The listing builds one solid part. Answer for the finished solid, in the listing's coordinates (mm). Face numbers are marked on the shaded views. A direction names the side the tool comes from. Round coordinates to 2 decimals unless told otherwise and drop trailing zeros. Order: outer loops, then holes, each group sorted by start corner. A loop starts at its lowest first (then second) coordinate and runs counter-clockwise, first axis right, second up. Notation, with made-up numbers: (74.5, 19.25) - (114.5, 19.25) arc R18 ccw to (114.5, 36.25) - close; hole circle Ø6 at (-32, 61.5). An arc over 180 degrees is marked (long way). Use CSV: the item, a comma, the result in double quotes. Start each with the question number.
Item 1: Find section C-C, the plane y = 29.5. Give the vertices of the cut face in (x, z), plus the area to 3 significant figures.
Item 2: Straight lines are drawn through the part: line 1 along X through (y, z) = (40, 0); line 2 along X through (y, z) = (2, -12.5); line 3 along X through (y, z) = (38.5, 6.5). For each, find the intervals that lie inside material, in ascending order. Write a range as [from, to].
Item 3: Flat-ended cylindrical pins translate along their axes: P1, Ø8, axis at x = -57, y = 34.5, coming from the -Z side; P2, Ø1.5, axis at x = -64.5, y = 41, coming from the +Z side; P3, Ø12, axis at y = 21, z = -34, coming from the +X side; P4, Ø9, axis at x = -61.25, z = 0, coming from the +Y side. Find the tip coordinate at first contact, or state that the pin passes through.
Item 4: Find section A-A, the plane x = 61.25. Give the vertices of the cut face in (y, z).
Item 5: Find section D-D, the plane y = 8. Give the vertices of the cut face in (x, z).
Item 6: For the marked faces 1, 2, 3, 4 and 5, determine the directions among +Z, -Z, +X, -X, +Y, -Y from which every point of the face is accessible in a straight line to the end or side of a thin tool.
Item 7: Find section B-B, the plane z = 0. Give the vertices of the cut face in (x, y).
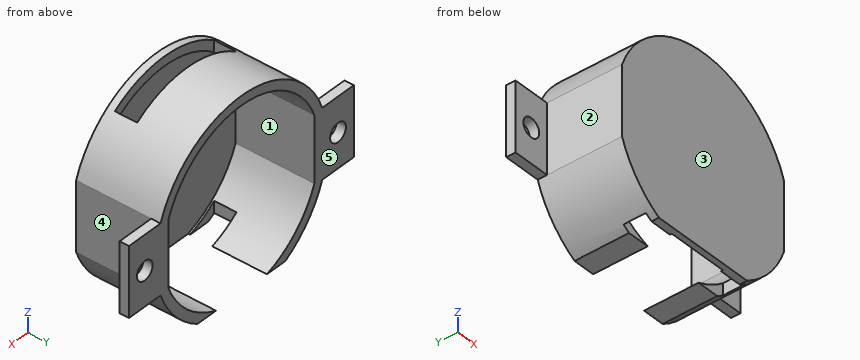
```python
from build123d import *

# Parameters (mm, degrees)
EXTRUDE_1_DEPTH          = 42.3
EXTRUDE_START            = 3
EXTRUDE_2_DEPTH          = 3
SKETCH_3_W               = 37.077621282
SKETCH_3_H               = 5
EXTRUDE_4_DEPTH          = 20
SKETCH_5_W               = 37.077621282
SKETCH_5_H               = 5
EXTRUDE_5_DEPTH          = 20
CUT_EXTRUDE_1_REACH      = 102.493
SKETCH_6_R               = 5
CUT_EXTRUDE_2_REACH      = 102.493
SKETCH_7_R               = 5
CUT_EXTRUDE_3_DEPTH      = 137.919145849
CUT_EXTRUDE_3_DEPTH_BACK = 137.919145849
SKETCH_9_W               = 62.954996742
SKETCH_9_H               = 12
CUT_EXTRUDE_4_DEPTH      = 101.493295796
CUT_EXTRUDE_4_DEPTH_BACK = 101.493295796
CUT_EXTRUDE_5_DEPTH      = 101.493295796
CUT_EXTRUDE_5_DEPTH_BACK = 101.493295796
SKETCH_11_W              = 70.692803697
SKETCH_11_H              = 7.082333279


with BuildPart() as part:
    # 草图1 → 凸台-拉伸1 (new body)
    with BuildSketch(Plane(origin=(0, 0, 0), x_dir=(1, 0, 0), z_dir=(0, 1, 0))):
        with BuildLine():
            Line((-51.25, 18.538810641), (-51.25, -18.538810641))
            ThreePointArc((-51.25, -18.538810641), (0, -54.5), (51.25, -18.538810641))
            Line((51.25, -18.538810641), (51.25, 18.538810641))
            ThreePointArc((51.25, 18.538810641), (0, 54.5), (-51.25, 18.538810641))
        make_face()
        with BuildLine():
            Line((-46.25, 17.640507362), (-46.25, -17.640507362))
            ThreePointArc((-46.25, -17.640507362), (0, -49.5), (46.25, -17.640507362))
            Line((46.25, -17.640507362), (46.25, 17.640507362))
            ThreePointArc((46.25, 17.640507362), (0, 49.5), (-46.25, 17.640507362))
        make_face(mode=Mode.SUBTRACT)
    extrude(amount=EXTRUDE_1_DEPTH)

    # 草图2 → 凸台-拉伸2 (add)
    with BuildSketch(Plane(origin=(0, 0, 0), x_dir=(-1, 0, 0), z_dir=(0, -1, 0)).offset(EXTRUDE_START)):
        with BuildLine():
            Line((51.25, -18.538810641), (51.25, 18.538810641))
            ThreePointArc((51.25, 18.538810641), (0, 54.5), (-51.25, 18.538810641))
            Line((-51.25, 18.538810641), (-51.25, -18.538810641))
            ThreePointArc((-51.25, -18.538810641), (0, -54.5), (51.25, -18.538810641))
        make_face()
    extrude(amount=-EXTRUDE_2_DEPTH)

    # 草图3 → 凸台-拉伸4 (add)
    with BuildSketch(Plane.ZY.offset(51.25)):
        with Locations((0, 39.8)):
            Rectangle(SKETCH_3_W, SKETCH_3_H)
    extrude(amount=EXTRUDE_4_DEPTH)

    # 草图5 → 凸台-拉伸5 (add)
    with BuildSketch(Plane(origin=(51.25, 0, 0), x_dir=(0, 0, -1), z_dir=(1, 0, 0))):
        with Locations((0, 39.8)):
            Rectangle(SKETCH_5_W, SKETCH_5_H)
    extrude(amount=EXTRUDE_5_DEPTH)

    # 草图6 → 切除-拉伸1 (cut, up to next)
    with BuildSketch(Plane(origin=(0, 42.3, 0), x_dir=(1, 0, 0), z_dir=(0, 1, 0)), mode=Mode.PRIVATE) as cut_extrude_1_sk1:
        with Locations(Location((-61.25, 0, 0), (0, 0, 270))):
            Circle(SKETCH_6_R)
    cut_extrude_1_tool1 = extrude(cut_extrude_1_sk1.sketch, amount=-CUT_EXTRUDE_1_REACH, mode=Mode.PRIVATE) & part.part
    add(cut_extrude_1_tool1.solids().sort_by_distance((-61.25, 42.3, 0))[0], mode=Mode.SUBTRACT)

    # 草图7 → 切除-拉伸2 (cut, up to next)
    with BuildSketch(Plane(origin=(0, 42.3, 0), x_dir=(1, 0, 0), z_dir=(0, 1, 0)), mode=Mode.PRIVATE) as cut_extrude_2_sk1:
        with Locations(Location((61.25, 0, 0), (0, 0, 270))):
            Circle(SKETCH_7_R)
    cut_extrude_2_tool1 = extrude(cut_extrude_2_sk1.sketch, amount=-CUT_EXTRUDE_2_REACH, mode=Mode.PRIVATE) & part.part
    add(cut_extrude_2_tool1.solids().sort_by_distance((61.25, 42.3, 0))[0], mode=Mode.SUBTRACT)

    # 草图9 → 切除-拉伸3 (cut, two sides: drawn at the far end of the back side and taken through both)
    with BuildSketch(Plane(origin=(0, 0, -54.5), x_dir=(-1, 0, 0), z_dir=(0, 0, -1)).offset(-CUT_EXTRUDE_3_DEPTH_BACK)):
        with Locations((0, 7)):
            Rectangle(SKETCH_9_W, SKETCH_9_H)
    extrude(amount=CUT_EXTRUDE_3_DEPTH + CUT_EXTRUDE_3_DEPTH_BACK, mode=Mode.SUBTRACT)

    # 草图10 → 切除-拉伸4 (cut, two sides: drawn at the far end of the back side and taken through both)
    with BuildSketch(Plane.XZ.offset(3).offset(-CUT_EXTRUDE_4_DEPTH_BACK)):
        with BuildLine():
            Line((21.685248442, -50), (-21.685248442, -50))
            ThreePointArc((-21.685248442, -50), (-11.073617375, -53.363142694), (-1.63e-07, -54.5))
            ThreePointArc((-1.63e-07, -54.5), (11.073617215, -53.363142728), (21.685248442, -50))
        make_face()
    extrude(amount=CUT_EXTRUDE_4_DEPTH + CUT_EXTRUDE_4_DEPTH_BACK, mode=Mode.SUBTRACT)

    # 草图11 → 切除-拉伸5 (cut, two sides: drawn at the far end of the back side and taken through both)
    with BuildSketch(Plane.XZ.offset(3).offset(-CUT_EXTRUDE_5_DEPTH_BACK)):
        with Locations((7.420622122, -50.342884842)):
            Rectangle(SKETCH_11_W, SKETCH_11_H)
    extrude(amount=CUT_EXTRUDE_5_DEPTH + CUT_EXTRUDE_5_DEPTH_BACK, mode=Mode.SUBTRACT)


solid = part.part
```
Worked out:
1,outline,"(-51.25, -18.54) arc R54.5 ccw to (-27.93, -46.8) - (-16.12, -46.8) arc R49.5 cw to (-46.25, -17.64) - (-46.25, 17.64) arc R49.5 cw to (46.25, 17.64) - (46.25, -17.64) arc R49.5 cw to (16.12, -46.8) - (27.93, -46.8) arc R54.5 ccw to (51.25, -18.54) - (51.25, 18.54) arc R54.5 ccw to (-51.25, 18.54) - close"
1,area,"1,390 mm²"
2,line 1,"x = [-71.25, -66.25], [-56.25, -46.25], [46.25, 56.25], [66.25, 71.25]"
2,line 2,"x = [-51.25, -46.25], [46.25, 51.25]"
2,line 3,"x = [-71.25, -46.25], [46.25, 71.25]"
3,P1,"stops at z = -18.54"
3,P2,"stops at z = 18.54"
3,P3,"stops at x = 46.76"
3,P4,"passes through"
4,outline,"(37.3, -18.54) - (42.3, -18.54) - (42.3, -5) - (37.3, -5) - close; (37.3, 5) - (42.3, 5) - (42.3, 18.54) - (37.3, 18.54) - close"
5,outline,"(-51.25, -18.54) arc R54.5 ccw to (-31.48, -44.49) - (-31.48, -38.2) arc R49.5 cw to (-46.25, -17.64) - (-46.25, 17.64) arc R49.5 cw to (-31.48, 38.2) - (-31.48, 44.49) arc R54.5 ccw to (-51.25, 18.54) - close; (31.48, -44.49) arc R54.5 ccw to (51.25, -18.54) - (51.25, 18.54) arc R54.5 ccw to (31.48, 44.49) - (31.48, 38.2) arc R49.5 cw to (46.25, 17.64) - (46.25, -17.64) arc R49.5 cw to (31.48, -38.2) - close"
6,face 1,"+Y"
6,face 2,"+Z, -Z, -X, -Y"
6,face 3,"+Z, -Z, +X, -X, -Y"
6,face 4,"+Z, -Z, +X, -Y"
6,face 5,"+Z, -Z, +X, -X, +Y"
7,outline,"(-71.25, 37.3) - (-66.25, 37.3) - (-66.25, 42.3) - (-71.25, 42.3) - close; (-56.25, 37.3) - (-51.25, 37.3) - (-51.25, -3) - (51.25, -3) - (51.25, 37.3) - (56.25, 37.3) - (56.25, 42.3) - (46.25, 42.3) - (46.25, 0) - (-46.25, 0) - (-46.25, 42.3) - (-56.25, 42.3) - close; (66.25, 37.3) - (71.25, 37.3) - (71.25, 42.3) - (66.25, 42.3) - close"
